Drawing for the job (mm, zero at the part's lowest x, y, z). Round coordinates to 2 decimals unless told otherwise and drop trailing zeros. Loops run counter-clockwise (first coordinate to the right, second up) from the corner with the lowest first, then second, coordinate; pieces in that order, holes last. Notation, with made-up numbers: M -40,-27.75 L -2,-27.75 A20 ccw -2,-18.75 Z; hole C 16.25,64 d6. An arc over 180 degrees is marked long. Use a Markdown table: item, result. Add a question column.
Q1. Cut at C-C (y = 2.1). Give the cut face in (x, z).
Q2. Cut at A-A (x = 5). Give the cut face in (y, z).
Q3. Probe line 1 (X direction, y = 0.7, z = 5); line 2 (Z direction, x = 125, y = 0.9); line 3 (X direction, y = 0.3, z = 18.5). List the from-to ranges inside material, lowest first. Write a range as from..to.
Q4. Pin check, flat tip, straight feed: pin 1 (2.5 mm diameter, centred on x = 5, z = 75, fed in from -Y). Stop position of the tip, or through.
Q5. Cut at D-D (x = 110). Give the cut face in (y, z).
Q6. Cut at B-B (z = 35). Give the cut face in (x, y), plus the area to 3 significant figures.
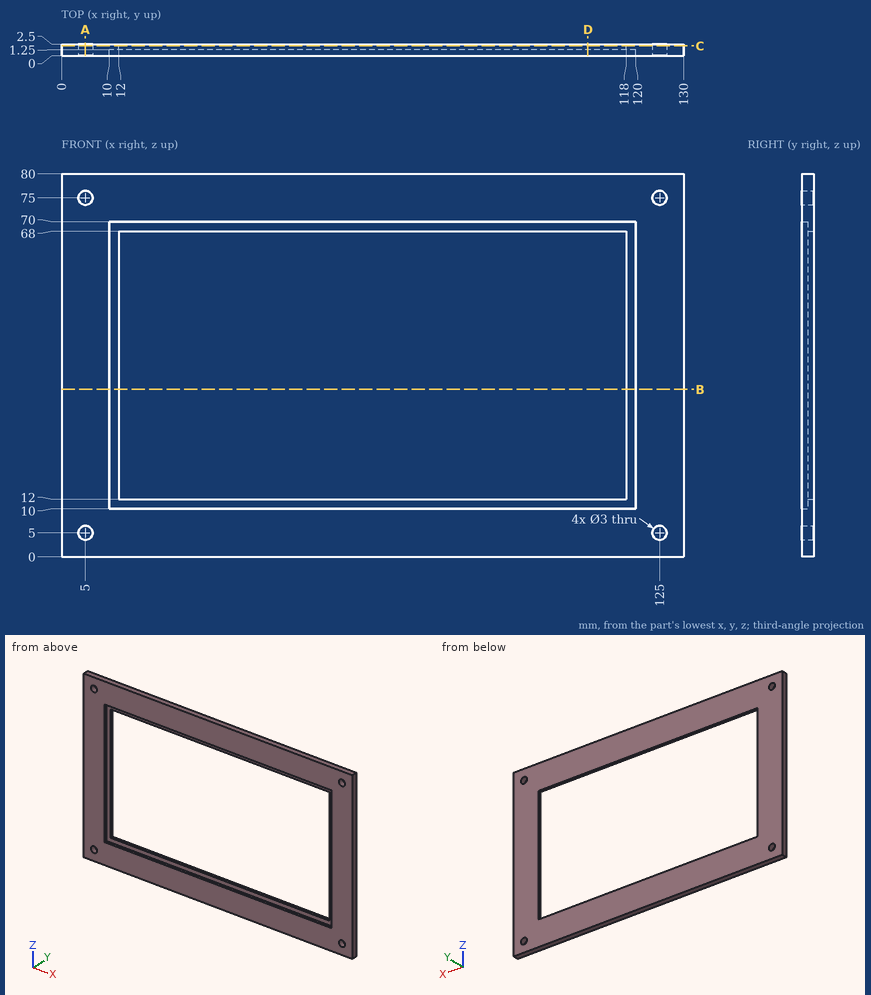
Checked values:
| question | item | result |
|---|---|---|
| 1 | outline | M 0,0 L 130,0 L 130,80 L 0,80 Z; hole C 5,5 d3; hole C 5,75 d3; hole M 12,12 L 118,12 L 118,68 L 12,68 Z; hole C 125,5 d3; hole C 125,75 d3 |
| 2 | outline | M 0,0 L 2.5,0 L 2.5,3.5 L 0,3.5 Z; M 0,6.5 L 2.5,6.5 L 2.5,73.5 L 0,73.5 Z; M 0,76.5 L 2.5,76.5 L 2.5,80 L 0,80 Z |
| 3 | line 1 | x = 0..3.5, 6.5..123.5, 126.5..130 |
| 3 | line 2 | z = 0..3.5, 6.5..73.5, 76.5..80 |
| 3 | line 3 | x = 0..10, 120..130 |
| 4 | pin 1 | passes through |
| 5 | outline | M 0,0 L 2.5,0 L 2.5,12 L 1.25,12 L 1.25,10 L 0,10 Z; M 0,70 L 1.25,70 L 1.25,68 L 2.5,68 L 2.5,80 L 0,80 Z |
| 6 | outline | M 0,0 L 10,0 L 10,1.25 L 12,1.25 L 12,2.5 L 0,2.5 Z; M 118,1.25 L 120,1.25 L 120,0 L 130,0 L 130,2.5 L 118,2.5 Z |
| 6 | area | 55.0 mm^2 |
